```python
from build123d import *

# Parameters (mm, degrees)
F0_W      = 74.689984
F0_H      = 131.0824
F1_DEPTH  = 37.31034
F1_FACE_W = 74.689984
F1_FACE_H = 131.0824
F2_DEPTH  = 34.998059
F3_T      = -2.54


with BuildPart() as f1:
    # F0 (on Top) → F1 (new body)
    with BuildSketch(Plane.XY):
        Rectangle(F0_W, F0_H)
    extrude(amount=F1_DEPTH)

    # F1_face (on face) → F2 (join)
    with BuildSketch(Plane(origin=(0, 0, 0), x_dir=(1, 0, 0), z_dir=(0, 0, -1))):
        Rectangle(F1_FACE_W, F1_FACE_H)
    extrude(amount=F2_DEPTH)

    # F3
    f3_openings = [f1.faces().sort_by_distance(p)[0] for p in [
        (0, -65.5412, 1.15614),
    ]]
    offset(amount=F3_T, openings=f3_openings)


solid = f1.part
```
Here's how the part is built. I have some questions about the finished solid (model axes, mm). A direction names the side the tool comes from. Round coordinates to 2 decimals unless told otherwise and drop trailing zeros. Loops run counter-clockwise (first coordinate to the right, second up) from the corner with the lowest first, then second, coordinate; pieces in that order, holes last. Notation, with made-up numbers: (-10, -28.5) -> (25, -28.5) arc R22 cw to (25, -17.5) -> close; hole circle Ø11 at (-25, 44). An arc over 180 degrees is marked (long way). Answer as CSV lines item,"result". Start each with the question number.
1. Imagine slicing it at A-A on y = -1. Write out the boundary of the cut face in (x, z) (3 decimals), plus the area to 3 significant figures.
2. I'm going to push a flat-ended pin straight in: P1, Ø2, axis at x = -22.5, z = -11, coming from the -Y side. Where does the tip first touch, or does it pass through?
3. Imagine slicing it at C-C on z = 21.5. Write out the boundary of the cut face in (x, y) (3 decimals).
4. Imagine slicing it at B-B on x = -12.5. Write out the boundary of the cut face in (y, z).
5. For faces 4 (the face through (-1, 1, 37.31)), 5 (the face through (0, 63.001, 2)), which set-ups out of +Z, -Z, +X, -X, +Y, -Y let a thin tool reach every point of the face, with its end or its side?
6. I need wall thicknesses on probe 1 along X at (y, z) = (-10.5, 18) (3 decimals); probe 2 along Z at (x, y) = (11.5, 45); probe 3 along Y at (x, z) = (17.5, 8). Which ranges of each line are inside material? Lowest first, please. Write a range as from..to.
7. If we mould it in two halves opening along Z, with no side actions, what happens to faces 1 (the face through (-1, -1, -34.998)), 2 (the face through (-3, -65.541, -33)), 3 (the face through (34.805, 0, 2))? For each: pulls with the +Z half, pulls with the -Z half, needs draft (parallel to the pull), parting line crosses it, or undercut.
Solution:
1,outline,"(-37.345, -34.998) -> (37.345, -34.998) -> (37.345, 37.31) -> (-37.345, 37.31) -> close; hole (-34.805, -32.458) -> (34.805, -32.458) -> (34.805, 34.77) -> (-34.805, 34.77) -> close"
1,area,"721 mm²"
2,P1,"y = 63"
3,outline,"(-37.345, -65.541) -> (-34.805, -65.541) -> (-34.805, 63.001) -> (34.805, 63.001) -> (34.805, -65.541) -> (37.345, -65.541) -> (37.345, 65.541) -> (-37.345, 65.541) -> close"
4,outline,"(-65.54, -35) -> (65.54, -35) -> (65.54, 37.31) -> (-65.54, 37.31) -> (-65.54, 34.77) -> (63, 34.77) -> (63, -32.46) -> (-65.54, -32.46) -> close"
5,face 4,"+Z, +X, -X, +Y, -Y"
5,face 5,"-Y"
6,probe 1,"-37.345..-34.805, 34.805..37.345"
6,probe 2,"-35..-32.46, 34.77..37.31"
6,probe 3,"63..65.54"
7,face 1,"pulls with the -Z half"
7,face 2,"needs draft"
7,face 3,"undercut"
